```python
from build123d import *

# Parameters (mm, degrees)
SKETCH1_R          = 34.925
EXTRUDE1_DEPTH     = 12.7
SKETCH2_R          = 19.05
CUT_EXTRUDE1_DEPTH = 13.7
SKETCH3_R          = 3.3655
CUT_EXTRUDE2_DEPTH = 13.7
CIRPATTERN1_COUNT  = 6


with BuildPart() as part:
    # Sketch1 → Extrude1 (new body)
    with BuildSketch(Plane(origin=(0, 0, 0), x_dir=(1, 0, 0), z_dir=(0, 1, 0))):
        Circle(SKETCH1_R)
    extrude(amount=EXTRUDE1_DEPTH)

    # Sketch2 → Cut-Extrude1 (cut, through all)
    with BuildSketch(Plane(origin=(0, 0, 0), x_dir=(1, 0, 0), z_dir=(0, 1, 0))):
        Circle(SKETCH2_R)
    extrude(amount=CUT_EXTRUDE1_DEPTH, mode=Mode.SUBTRACT)

    # Sketch3 → Cut-Extrude2 (cut, through all)
    with BuildSketch(Plane(origin=(0, 0, 0), x_dir=(1, 0, 0), z_dir=(0, 1, 0))):
        with Locations((0, 29.337)):
            Circle(SKETCH3_R)
    cut_extrude2 = extrude(amount=CUT_EXTRUDE2_DEPTH, mode=Mode.SUBTRACT)

    # CirPattern1: Cut-Extrude2 ×6 about axis
    cirpattern1_axis = Axis((0, 0, 0), (0, 1, 0))
    for i in range(1, CIRPATTERN1_COUNT):
        add(cut_extrude2.rotate(cirpattern1_axis, i * 360 / CIRPATTERN1_COUNT), mode=Mode.SUBTRACT)


solid = part.part
```
Design review of the part built by this model. Coordinates are the model's own, in mm. Round coordinates to 2 decimals unless told otherwise and drop trailing zeros. Order: outer loops, then holes, each group sorted by start corner. A loop starts at its lowest first (then second) coordinate and runs counter-clockwise, first axis right, second up. Notation, with made-up numbers: (-3, -25.5) - (36, -25.5) arc R20 cw to (36, 0.5) - close; hole circle Ø7 at (0.5, 63.25). An arc over 180 degrees is marked (long way). Return JSON: item names as keys, results as strings.
Q1. Consider section A-A on z = 0. Write out the cut boundary in (x, y) (3 decimals).
Computed values:
{"outline": "(-34.925, 0) - (-19.05, 0) - (-19.05, 12.7) - (-34.925, 12.7) - close; (19.05, 0) - (34.925, 0) - (34.925, 12.7) - (19.05, 12.7) - close"}
Q2. The part is to be moulded in two halves that separate along Z. For faces 1 (the cylindrical face through (-15.12, 6.26, 11.59)), 2 (the flat face through (15, 0, 15)), 3 (the cylindrical face through (-27.715, 6.261, 21.251)), say which applies: pulls with the +Z half, pulls with the -Z half, needs draft (parallel to the pull), parting line crosses it, or undercut.
Computed values:
{"face 1": "undercut", "face 2": "needs draft", "face 3": "parting line crosses it"}
Q3. Consider section B-B on x = 0. Give the number of separate pieces and of enclosed holes in the cut face, plus the area to 3 significant figures.
Computed values:
{"separate pieces": "4", "enclosed holes": "0", "area": "232 mm2"}
Q4. Wall thickness on L1, parallel to X at y = 2.5, z = 13; L2, parallel to Z at x = 27, y = 4; L3, parallel to Z at x = 25.5, y = 1.5: over which ranges is each line inside the solid? List them lowest first. Write a range as [from, to].
Computed values:
{"L1": "x = [-32.42, -28.33], [-22.48, -13.92], [13.92, 22.48], [28.33, 32.42]", "L2": "z = [-22.15, -17.63], [-11.7, 11.7], [17.63, 22.15]", "L3": "z = [-23.86, -18.03], [-11.3, 11.3], [18.03, 23.86]"}
Q5. For pin 1 Ø1.5 at (x, z) = (26, -12.5) entering from +Y; pin 2 Ø3 at (x, y) = (-20.5, 2) entering from -Z; pin 3 Ø1.5 at (y, z) = (8, 7) entering from -X; pin 4 Ø1.5 at (y, z) = (5.5, -25) entering from +X, all flat-tipped, find the tip position at first contact; note any pin that passes through.
Computed values:
{"pin 1": "passes through", "pin 2": "stops at z = -29.3", "pin 3": "stops at x = -34.36", "pin 4": "stops at x = 25.13"}
Q6. Consider section C-C on x = -25. Write out the cut boundary in (y, z).
Computed values:
{"outline": "(0, -24.39) - (12.7, -24.39) - (12.7, -18.01) - (0, -18.01) - close; (0, -11.33) - (12.7, -11.33) - (12.7, 11.33) - (0, 11.33) - close; (0, 18.01) - (12.7, 18.01) - (12.7, 24.39) - (0, 24.39) - close"}
